Input: part model. Units: mm. Frame: model coordinates. A direction names the side the tool comes from. Round coordinates to 2 decimals unless told otherwise and drop trailing zeros. Order: outer loops, then holes, each group sorted by start corner. A loop starts at its lowest first (then second) coordinate and runs counter-clockwise, first axis right, second up. Notation, with made-up numbers: (-18, 75.5) -> (10, 75.5) arc R36 cw to (10, 111.5) -> close; hole circle Ø9 at (43, 24). An arc over 180 degrees is marked (long way). Answer as CSV lines item,"result". Start each with the question number.
1) First-contact query: P1, Ø0.8, axis at y = 1, z = -2.5, coming from the -X side. Flat tip, straight axial feed; report the tip coordinate or a pass-through.
2) Mould query, pull axis X, two halves, no side actions, for faces 4 (the face through (0.955, 1, -2)), 5 (the face through (-1, 1, -1.4)), 6 (the face through (-3.4, 1, 0)). Classes: +X half, -X half, draft (parallel to the pull), parting line (faces both ways), or undercut.
3) Line query: L1, parallel to Y at x = 2.25, z = -0.95; L2, parallel to Z at x = 1.5, y = 0.4; L3, parallel to Z at x = 0.25, y = 1. Output: solid intervals per line, ascending.
4) Section query D-D, the plane x = -3. Output: boundary loops of the cut face in (y, z).
5) Access query for faces 1 (the face through (-0.445, 1, -2)), 2 (the face through (0, 0.35, -2)), 3 (the face through (3.4, 1, 0)). Directions: +Z, -Z, +X, -X, +Y, -Y. A direction counts if a zero-diameter tool reaches every point of the face in a straight line with its end or side. Return the directions, or none.
6) Section query B-B, the plane y = 0.6. Output: boundary loops of the cut face in (x, z), and give its area (3 significant figures).
7) Section query A-A, the plane z = 2.05. Output: boundary loops of the cut face in (x, y), and give its area (3 significant figures).
```python
from build123d import *

# Parameters (mm, degrees)
SKETCH1_W             = 6.8
SKETCH1_H             = 2.8
BOSS_EXTRUDE1_DEPTH   = 1.4
BOSS_EXTRUDE2_DEPTH   = 2.8
BOSS_EXTRUDE2_2_DEPTH = 2.8
BOSS_EXTRUDE3_DEPTH   = 2.8
CUT_EXTRUDE1_DEPTH    = 1.1
SKETCH8_W             = 0.2
SKETCH8_H             = 1
BOSS_EXTRUDE4_DEPTH   = 0.15
SKETCH9_W             = 1.4
SKETCH9_H             = 1.05
BOSS_EXTRUDE5_DEPTH   = 1.51


with BuildPart() as part:
    # Sketch1 → Boss-Extrude1 (new body)
    with BuildSketch(Plane(origin=(0, 0, 0), x_dir=(1, 0, 0), z_dir=(0, 1, 0))):
        Rectangle(SKETCH1_W, SKETCH1_H)
    extrude(amount=BOSS_EXTRUDE1_DEPTH)



with BuildPart() as body_2:
    # Sketch3 → Boss-Extrude2 (new body)
    with BuildSketch(Plane.XY.offset(1.4)):
        with BuildLine():
            Line((-3.9, 0), (-3.687815007, 0))
            ThreePointArc((-3.687815007, 0), (-3.58174899, 0.043933983), (-3.537815007, 0.15))
            Line((-3.537815007, 0.15), (-3.537815007, 1.44554352))
            Line((-3.537815007, 1.44554352), (-2.932940076, 1.44554352))
            Line((-2.932940076, 1.44554352), (-2.932940076, 1.641087041))
            Line((-2.932940076, 1.641087041), (-3.424164264, 1.641087041))
            ThreePointArc((-3.424164264, 1.641087041), (-3.636296298, 1.553219075), (-3.724164264, 1.341087041))
            Line((-3.724164264, 1.341087041), (-3.724164264, 0.25))
            ThreePointArc((-3.724164264, 0.25), (-3.753453586, 0.179289322), (-3.824164264, 0.15))
            Line((-3.824164264, 0.15), (-3.9, 0.15))
            Line((-3.9, 0.15), (-3.9, 0))
        make_face()
    extrude(amount=-BOSS_EXTRUDE2_DEPTH)


with BuildPart() as body_3:
    # Sketch3 → Boss-Extrude2 2 (new body)
    with BuildSketch(Plane.XY.offset(1.4)):
        with BuildLine():
            Line((3.824164264, 0.15), (3.9, 0.15))
            Line((3.9, 0.15), (3.9, 0))
            Line((3.9, 0), (3.687815007, 0))
            ThreePointArc((3.687815007, 0), (3.58174899, 0.043933983), (3.537815007, 0.15))
            Line((3.537815007, 0.15), (3.537815007, 1.44554352))
            Line((3.537815007, 1.44554352), (2.932940076, 1.44554352))
            Line((2.932940076, 1.44554352), (2.932940076, 1.641087041))
            Line((2.932940076, 1.641087041), (3.424164264, 1.641087041))
            ThreePointArc((3.424164264, 1.641087041), (3.636296298, 1.553219075), (3.724164264, 1.341087041))
            Line((3.724164264, 1.341087041), (3.724164264, 0.25))
            ThreePointArc((3.724164264, 0.25), (3.753453586, 0.179289322), (3.824164264, 0.15))
        make_face()
    extrude(amount=-BOSS_EXTRUDE2_2_DEPTH)


with BuildPart() as part_1:
    add(part.part)

    add(body_2.part)  # Boss-Extrude3 merges body 2

    add(body_3.part)  # Boss-Extrude3 merges body 3
    # Sketch4 → Boss-Extrude3 (add)
    with BuildSketch(Plane.XY.offset(1.4)):
        Polygon((-2.805997344, 1.4), (-2.805997344, 1.644514916), (-2.905997344, 1.744514916), (-3.226717158, 1.744514916), (-3.38829441, 1.665722517), (-3.621220366, 1.367677477), (-3.582797618, 1.288885079), (-2.805997344, 1.288885079), align=None)
        Polygon((3.582797618, 1.288885079), (2.805997344, 1.288885079), (2.805997344, 1.4), (2.805997344, 1.644514916), (2.905997344, 1.744514916), (3.226717158, 1.744514916), (3.38829441, 1.665722517), (3.621220366, 1.367677477), align=None)
    extrude(amount=-BOSS_EXTRUDE3_DEPTH)

    # Sketch6 → Cut-Extrude1 (cut, symmetric)
    with BuildSketch(Plane.XY):
        with BuildLine():
            Line((-3.537815007, 1.288885079), (-3.724164264, 1.288885079))
            Line((-3.724164264, 1.288885079), (-3.724164264, 0.25))
            ThreePointArc((-3.724164264, 0.25), (-3.753453586, 0.179289322), (-3.824164264, 0.15))
            Line((-3.824164264, 0.15), (-3.9, 0.15))
            Line((-3.9, 0.15), (-3.9, 0))
            Line((-3.9, 0), (-3.687815007, 0))
            ThreePointArc((-3.687815007, 0), (-3.58174899, 0.043933983), (-3.537815007, 0.15))
            Line((-3.537815007, 0.15), (-3.537815007, 1.288885079))
        make_face()
        with BuildLine():
            Line((3.537815007, 1.288885079), (3.724164264, 1.288885079))
            Line((3.724164264, 1.288885079), (3.724164264, 0.25))
            ThreePointArc((3.724164264, 0.25), (3.753453586, 0.179289322), (3.824164264, 0.15))
            Line((3.824164264, 0.15), (3.9, 0.15))
            Line((3.9, 0.15), (3.9, 0))
            Line((3.9, 0), (3.687815007, 0))
            ThreePointArc((3.687815007, 0), (3.58174899, 0.043933983), (3.537815007, 0.15))
            Line((3.537815007, 0.15), (3.537815007, 1.288885079))
        make_face()
    extrude(amount=CUT_EXTRUDE1_DEPTH, both=True, mode=Mode.SUBTRACT)

    # Sketch8 → Boss-Extrude4 (add)
    with BuildSketch(Plane.XZ):
        with Locations((-1.8, 1.9)):
            Rectangle(SKETCH8_W, SKETCH8_H)
        with Locations((1.2, 1.9)):
            Rectangle(SKETCH8_W, SKETCH8_H)
        with Locations((2.7, 1.9)):
            Rectangle(SKETCH8_W, SKETCH8_H)
    extrude(amount=-BOSS_EXTRUDE4_DEPTH)

    # Sketch9 → Boss-Extrude5 (add)
    with BuildSketch(Plane(origin=(0, 0, -1.4), x_dir=(-1, 0, 0), z_dir=(0, 0, -1))):
        with Locations((-0.254692735, 0.875)):
            Rectangle(SKETCH9_W, SKETCH9_H)
    extrude(amount=BOSS_EXTRUDE5_DEPTH)


solid = part_1.part
```
Findings:
1,P1,"stops at x = -0.45"
2,face 4,"+X half"
2,face 5,"draft"
2,face 6,"undercut"
3,L1,"y = 0 to 1.4"
3,L2,"z = -1.4 to 1.4"
3,L3,"z = -2.91 to 1.4"
4,outline,"(0, -1.4) -> (1.74, -1.4) -> (1.74, 1.4) -> (0, 1.4) -> close"
5,face 1,"-Z, -X, +Y, -Y"
5,face 2,"-Z, +X, -X, -Y"
5,face 3,"+Z, -Z, -Y"
6,outline,"(-3.72, -1.4) -> (-3.54, -1.4) -> (-3.54, -1.1) -> (-3.72, -1.1) -> close; (-3.72, 1.1) -> (-3.54, 1.1) -> (-3.54, 1.4) -> (-3.72, 1.4) -> close; (-3.4, -1.4) -> (-0.45, -1.4) -> (-0.45, -2.91) -> (0.95, -2.91) -> (0.95, -1.4) -> (3.4, -1.4) -> (3.4, 1.4) -> (-3.4, 1.4) -> close; (3.54, -1.4) -> (3.72, -1.4) -> (3.72, -1.1) -> (3.54, -1.1) -> close; (3.54, 1.1) -> (3.72, 1.1) -> (3.72, 1.4) -> (3.54, 1.4) -> close"
6,area,"21.4 mm^2"
7,outline,"(-1.9, 0) -> (-1.7, 0) -> (-1.7, 0.15) -> (-1.9, 0.15) -> close; (1.1, 0) -> (1.3, 0) -> (1.3, 0.15) -> (1.1, 0.15) -> close; (2.6, 0) -> (2.8, 0) -> (2.8, 0.15) -> (2.6, 0.15) -> close"
7,area,"0.0900 mm^2"
